Check sheet for the modelled part. Datum: model origin and axes. Units: mm. Face numbers are marked on the shaded views. Round coordinates to 2 decimals unless told otherwise and drop trailing zeros. Order: outer loops, then holes, each group sorted by start corner. A loop starts at its lowest first (then second) coordinate and runs counter-clockwise, first axis right, second up.
Q1. Depth check by flat-ended pin: P1, Ø6, axis at x = 36, y = -42, coming from the -Z side; P2, Ø4, axis at x = 25, y = 26.5, coming from the +Z side; P3, Ø8, axis at x = -28, y = 37.5, coming from the +Z side. Enter the tip coordinate at first touch or a pass-through.
Q2. Mould release check, pull along Y, two halves, no side actions. Record for the marked faces 1 and 2: +Y half, -Y half, draft (parallel to the pull), parting line (faces both ways), or undercut.
Q3. Cross-section at A-A on y = 0. Record the cut outline in (x, z).
Q4. Cross-section at C-C on z = 1.95. Record the cut outline in (x, y), then the cut area to 3 significant figures.
Q5. Scan lines: probe 1 along Y at (x, z) = (0, 2.8); probe 2 along Y at (x, z) = (0, 4.15); probe 3 along Z at (x, y) = (14.5, -30.5). Record each from-to range of solid material in increasing order.
from build123d import *


with BuildPart() as part:
    # Sketch → Revolution (revolve)
    with BuildSketch(Plane.XZ):
        with BuildLine():
            Line((0, 0), (52.25, 0))
            ThreePointArc((52.25, 0), (52.603553, 0.146447), (52.75, 0.5))
            Line((52.75, 4.3), (52.75, 0.5))
            ThreePointArc((52.75, 4.3), (52.603553, 4.653553), (52.25, 4.8))
            Line((50.85, 4.8), (52.25, 4.8))
            ThreePointArc((50.85, 4.8), (50.496447, 4.653553), (50.35, 4.3))
            Line((50.35, 3.8), (50.35, 4.3))
            Line((50.75, 3.8), (50.35, 3.8))
            Line((50.75, 0.8), (50.75, 3.8))
            Line((0, 0.8), (50.75, 0.8))
            Line((0, 0), (0, 0.8))
        make_face()
    revolve(axis=Axis((0, 0, 0), (0, 0, 1)))


solid = part.part
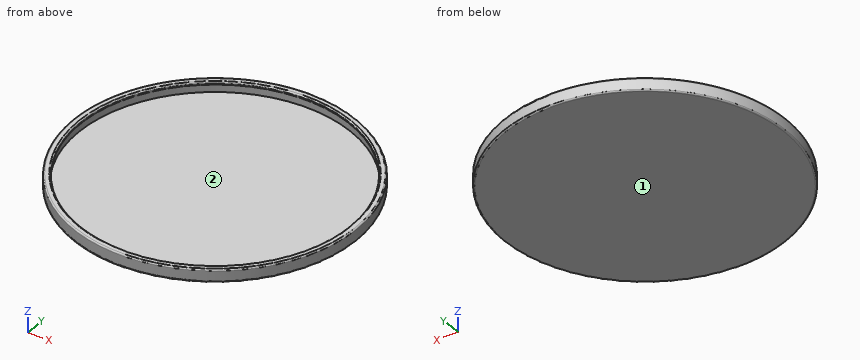
Results found:
1. P1: stops at z = 0
1. P2: stops at z = 0.8
1. P3: stops at z = 4.8
2. face 1: draft
2. face 2: undercut
3. outline: (-52.75, 0.5) arc R0.5 ccw to (-52.25, 0) - (52.25, 0) arc R0.5 ccw to (52.75, 0.5) - (52.75, 4.3) arc R0.5 ccw to (52.25, 4.8) - (50.85, 4.8) arc R0.5 ccw to (50.35, 4.3) - (50.35, 3.8) - (50.75, 3.8) - (50.75, 0.8) - (-50.75, 0.8) - (-50.75, 3.8) - (-50.35, 3.8) - (-50.35, 4.3) arc R0.5 ccw to (-50.85, 4.8) - (-52.25, 4.8) arc R0.5 ccw to (-52.75, 4.3) - close
4. outline: circle Ø105.5 at (0, 0); hole circle Ø101.5 at (0, 0)
4. area: 650 mm2
5. probe 1: y = -52.75 to -50.75, 50.75 to 52.75
5. probe 2: y = -52.75 to -50.35, 50.35 to 52.75
5. probe 3: z = 0 to 0.8
